Can you work these out from the drawing? Everything is in mm from the part's minimum corner. A direction names the side the tool comes from. Round coordinates to 2 decimals unless told otherwise and drop trailing zeros. Write each loop counter-clockwise with the first axis right and the second up, starting at its lowest first coordinate (ties: lowest second). Pieces come first, ordered by that corner, then holes.
Q1. If we section it at B-B (x = 6): Please give me the cut outline in (y, z).
Q2. If we section it at C-C (z = 4): Please give me the cut outline in (x, y), plus the area to 3 significant figures.
Q3. For the marked faces 1 and 2, which set-ups out of +Z, -Z, +X, -X, +Y, -Y let a thin tool reach every point of the face, with its end or its side?
Q4. Please list where these lines run through material, in increasing order: line 1 along Y through (x, z) = (6, 12.75); line 2 along Z through (x, y) = (7.5, 7.5).
Q5. I'm going to push flat-ended pins straight in: pin 1 Ø1.5 at (x, y) = (11.5, 8.5) entering from +Z; pin 2 Ø1 at (y, z) = (11, 9) entering from -X; pin 3 Ø1 at (y, z) = (2, 7) entering from +X. Where does each tip first touch, or does it pass through?
Q6. If we section it at D-D (x = 7.5): Please give me the cut outline in (y, z).
Q7. If we section it at A-A (z = 7.5): Please give me the cut outline in (x, y).
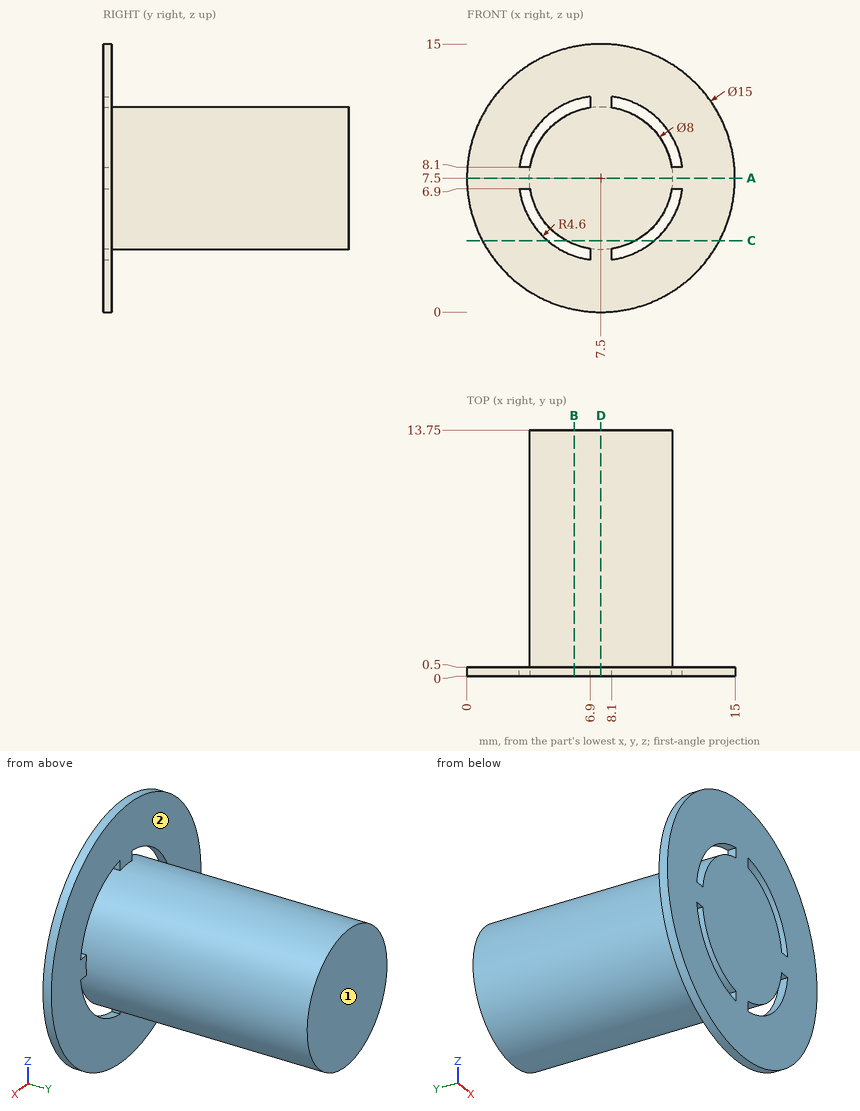
A:
1. outline: (0, 0.15) - (0.5, 0.15) - (0.5, 3.15) - (0, 3.15) - close; (0, 3.79) - (13.75, 3.79) - (13.75, 11.21) - (0, 11.21) - close; (0, 11.85) - (0.5, 11.85) - (0.5, 14.85) - (0, 14.85) - close
2. outline: (0.87, 0) - (4.52, 0) - (4.52, 0.5) - (0.87, 0.5) - close; (5.56, 0) - (9.44, 0) - (9.44, 13.75) - (5.56, 13.75) - close; (10.48, 0) - (14.13, 0) - (14.13, 0.5) - (10.48, 0.5) - close
2. area: 56.9 mm2
3. face 1: +Z, -Z, +X, -X, +Y
3. face 2: +Y
4. line 1: y = 0 to 0.5
4. line 2: z = 3.5 to 11.5
5. pin 1: stops at z = 9.83
5. pin 2: stops at x = 3.63
5. pin 3: stops at x = 11.5
6. outline: (0, 0) - (0.5, 0) - (0.5, 3.5) - (13.75, 3.5) - (13.75, 11.5) - (0.5, 11.5) - (0.5, 15) - (0, 15) - close
7. outline: (0, 0) - (15, 0) - (15, 0.5) - (11.5, 0.5) - (11.5, 13.75) - (3.5, 13.75) - (3.5, 0.5) - (0, 0.5) - close
